from build123d import *

# Parameters (mm, degrees)
SKETCH1_W            = 94
SKETCH1_H            = 130
BOSS_EXTRUDE1_DEPTH  = 23
SKETCH3_W            = 24
SKETCH3_H            = 6
BOSS_EXTRUDE2_DEPTH  = 6
SKETCH4_W            = 6
SKETCH4_H            = 5
CUT_EXTRUDE1_DEPTH   = 2
SKETCH5_W            = 5
SKETCH5_H            = 5
CUT_EXTRUDE2_DEPTH   = 18
LPATTERN1_COUNT      = 2
LPATTERN1_PITCH      = 69
LPATTERN1_COUNT_DIR2 = 2
LPATTERN1_PITCH_DIR2 = 115
FILLET1_R            = 2
SKETCH6_R            = 4
CUT_EXTRUDE3_DEPTH   = 7


with BuildPart() as part:
    # Sketch1 → Boss-Extrude1 (new body)
    with BuildSketch(Plane(origin=(0, 0, 0), x_dir=(1, 0, 0), z_dir=(0, 1, 0))):
        with Locations((47, 65)):
            Rectangle(SKETCH1_W, SKETCH1_H)
        Polygon((79, 125), (79, 120), (89, 120), (89, 10), (79, 10), (79, 5), (15, 5), (15, 10), (5, 10), (5, 120), (15, 120), (15, 125), align=None, mode=Mode.SUBTRACT)
    extrude(amount=BOSS_EXTRUDE1_DEPTH)

    # Sketch3 → Boss-Extrude2 (add)
    with BuildSketch(Plane(origin=(5, 0, 0), x_dir=(0, 0, -1), z_dir=(1, 0, 0))):
        with Locations((100, 18.5)):
            Rectangle(SKETCH3_W, SKETCH3_H)
    boss_extrude2 = extrude(amount=BOSS_EXTRUDE2_DEPTH)

    # Mirror3: Boss-Extrude2 across plane
    add(boss_extrude2.mirror(Plane.ZY.offset(-47)))

    # Sketch4 → Cut-Extrude1 (cut)
    with BuildSketch(Plane(origin=(0, 21.5, 0), x_dir=(1, 0, 0), z_dir=(0, 1, 0))):
        with Locations((86, 100)):
            Rectangle(SKETCH4_W, SKETCH4_H)
    extrude(amount=-CUT_EXTRUDE1_DEPTH, mode=Mode.SUBTRACT)

    # Sketch5 → Cut-Extrude2 (cut)
    with BuildSketch(Plane.XZ):
        with Locations((81.5, -122.5)):
            Rectangle(SKETCH5_W, SKETCH5_H)
    cut_extrude2 = extrude(amount=-CUT_EXTRUDE2_DEPTH, mode=Mode.SUBTRACT)

    # LPattern1: Cut-Extrude2 2 × 2
    with Locations(*[(-i * LPATTERN1_PITCH, 0, j * LPATTERN1_PITCH_DIR2) for i in range(LPATTERN1_COUNT) for j in range(LPATTERN1_COUNT_DIR2) if (i, j) != (0, 0)]):
        add(cut_extrude2, mode=Mode.SUBTRACT)

    # Fillet1
    fillet1_edges = [part.edges().sort_by_distance(p)[0] for p in [
        (0, 11.5, -130),
        (94, 11.5, -130),
        (94, 11.5, 0),
        (0, 11.5, 0),
    ]]
    fillet(fillet1_edges, radius=FILLET1_R)

    # Sketch6 → Cut-Extrude3 (cut)
    with BuildSketch(Plane.XY):
        with Locations((22, 10)):
            Circle(SKETCH6_R)
    extrude(amount=-CUT_EXTRUDE3_DEPTH, mode=Mode.SUBTRACT)


solid = part.part
Build history of the part. All positions in model axes, mm. A direction names the side the tool comes from. Round coordinates to 2 decimals unless told otherwise and drop trailing zeros. Write each loop counter-clockwise with the first axis right and the second up, starting at its lowest first coordinate (ties: lowest second). Pieces come first, ordered by that corner, then holes. Notation, with made-up numbers: (-27.75, 79.25) -> (-10.75, 79.25) arc R20 cw to (-10.75, 110.25) -> close; hole circle Ø4 at (-30.5, -24.75). An arc over 180 degrees is marked (long way). Use one line per item in the form item = value.
Q1. Band-saw the part on A-A, the plane x = 22. Write the cut outline in (y, z), then the cut area to 3 significant figures.
Conclusion:
outline = (0, -130) -> (23, -130) -> (23, -125) -> (0, -125) -> close; (0, -5) -> (6, -5) -> (6, 0) -> (0, 0) -> close; (14, -5) -> (23, -5) -> (23, 0) -> (14, 0) -> close
area = 190 mm²
Q2. Band-saw the part on C-C, the plane y = 1.5. Write the cut outline in (x, z), then the cut area to 3 significant figures.
Conclusion:
outline = (0, -128) arc R2 ccw to (2, -130) -> (92, -130) arc R2 ccw to (94, -128) -> (94, -2) arc R2 ccw to (92, 0) -> (2, 0) arc R2 ccw to (0, -2) -> close; hole (5, -120) -> (10, -120) -> (10, -125) -> (84, -125) -> (84, -120) -> (89, -120) -> (89, -10) -> (84, -10) -> (84, -5) -> (10, -5) -> (10, -10) -> (5, -10) -> close
area = 2,240 mm²
Q3. Band-saw the part on B-B, the plane z = -92.5. Write the cut outline in (x, y).
Conclusion:
outline = (0, 0) -> (5, 0) -> (5, 15.5) -> (11, 15.5) -> (11, 21.5) -> (5, 21.5) -> (5, 23) -> (0, 23) -> close; (83, 15.5) -> (89, 15.5) -> (89, 0) -> (94, 0) -> (94, 23) -> (89, 23) -> (89, 21.5) -> (83, 21.5) -> close
Q4. Band-saw the part on D-D, the plane x = 74.5. Write the cut outline in (y, z).
Conclusion:
outline = (0, -130) -> (23, -130) -> (23, -125) -> (0, -125) -> close; (0, -5) -> (23, -5) -> (23, 0) -> (0, 0) -> close
Q5. Tool access for faces 4 (the flat face through (86, 21.5, -107)), 5 (the flat face through (86, 18, -112)), 6 (the flat face through (12, 18, -122)), 7 (the cylindrical face through (18, 10, -2)), 8 (the flat face through (2, 0, -65)): list every direction of +Z, -Z, +X, -X, +Y, -Y with a clear straight run to the whole face (end or side of a thin tool).
Conclusion:
face_4 = +Y
face_5 = +Y, -Y
face_6 = -Y
face_7 = +Z
face_8 = +Z, -Z, +X, -X, -Y
Q6. Drop a flat-ended pin along its axis: P1, Ø4, axis at x = 13, z = -8.5, coming from the -Y side. Give the stop position or say it passes through.
Conclusion:
P1 = 18
Q7. Drill centre lines: L1, parallel to Z at x = 70.5, y = 3.5; L2, parallel to X at y = 1.25, z = -47; L3, parallel to Y at x = 22, z = -1.9. Where is each one in solid material? Low to high.
Conclusion:
L1 = -130 to -125, -5 to 0
L2 = 0 to 5, 89 to 94
L3 = 0 to 6, 14 to 23
Q8. Two-plate mould, pull along Z, no slides. Class faces 1 (the flat face through (46, 11, 0)), 2 (the flat face through (8, 18, -88)), 3 (the flat face through (94, 11, -64)): released by +Z, released by -Z, zero draft, split by the parting line, or undercut.
Conclusion:
face_1 = released by +Z
face_2 = undercut
face_3 = zero draft
